Input: dimensioned drawing with shaded views. Units: mm. Origin: part minimum x, y, z. A direction names the side the tool comes from. Round coordinates to 2 decimals unless told otherwise and drop trailing zeros. Loops run counter-clockwise (first coordinate to the right, second up) from the corner with the lowest first, then second, coordinate; pieces in that order, holes last. Notation, with made-up numbers: (-13, 51) - (-1, 51) arc R22 cw to (-1, 84) - close; hole circle Ø9 at (2, 54.25). An arc over 180 degrees is marked (long way). Answer as a JSON object with one key per item and string values. Group by question number.
Item 1: Section B-B (y = 12.75). Return the cut outline in (x, z) (1 decimal), plus the area to 3 significant figures.
Item 2: Line query: line 1 (Y direction, x = 8, z = 133.5); line 2 (X direction, y = 8.5, z = 24); line 3 (Z direction, x = 15.5, y = 12.75) (1 decimal). Output: solid intervals per line, ascending.
Item 3: Reachability of the marked faces 1, 2 and 3 from +Z, -Z, +X, -X, +Y, -Y: full face, straight path, thin tool, end or side. Return the list, or none.
Item 4: Section C-C (z = 96). Return the cut outline in (x, y).
Item 5: Section D-D (y = 7). Return the cut outline in (x, z).
Item 6: First-contact query: pin 1 (1.4 mm diameter, centred on x = 6.12, z = 127.1, fed in from +Y); pin 2 (5.5 mm diameter, centred on x = 6, z = 47, fed in from +Y); pin 3 (8 mm diameter, centred on x = 8.5, y = 10, fed in from +Z); pin 4 (1.4 mm diameter, centred on x = 21.5, y = 13.5, fed in from -Z) (1 decimal). Flat tips, straight axial feed; report the tip coordinate or a pass-through.
Item 7: Section A-A (x = 39). Return the cut outline in (y, z) (1 decimal).
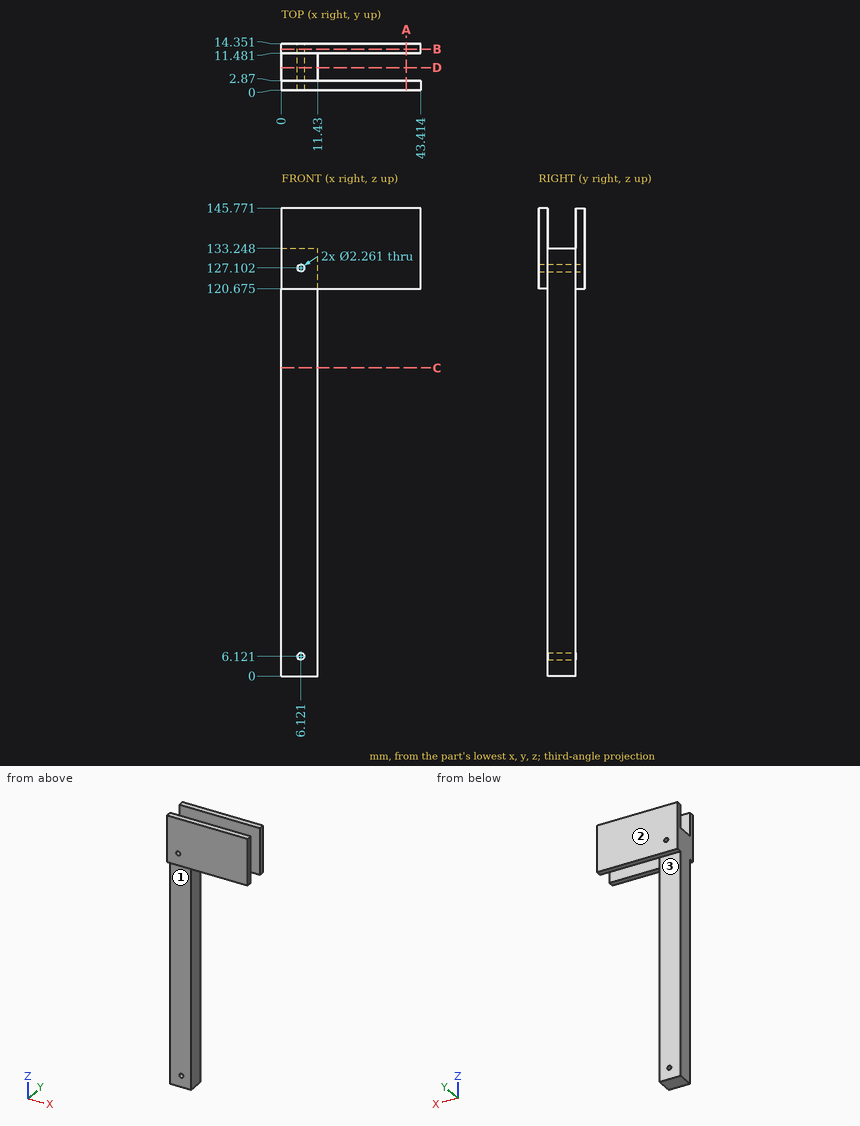
Values:
{
 "1": {"outline": "(0, 120.7) - (43.4, 120.7) - (43.4, 145.8) - (0, 145.8) - close; hole circle Ø2.3 at (6.1, 127.1)", "area": "1,090 mm^2"},
 "2": {"line 1": "y = 0 to 2.87, 11.48 to 14.35", "line 2": "x = 0 to 11.43", "line 3": "z = 120.7 to 145.8"},
 "3": {"face 1": "-Z, +X, -X, -Y", "face 2": "+Z, -Z, +X, -X, +Y", "face 3": "-Z, +X, -X, +Y"},
 "4": {"outline": "(0, 2.87) - (11.43, 2.87) - (11.43, 11.48) - (0, 11.48) - close"},
 "5": {"outline": "(0, 0) - (11.43, 0) - (11.43, 133.25) - (0, 133.25) - close; hole circle Ø2.26 at (6.12, 6.12); hole circle Ø2.26 at (6.12, 127.1)"},
 "6": {"pin 1": "passes through", "pin 2": "stops at y = 11.48", "pin 3": "stops at z = 145.77", "pin 4": "stops at z = 120.7"},
 "7": {"outline": "(0, 120.7) - (2.9, 120.7) - (2.9, 145.8) - (0, 145.8) - close; (11.5, 120.7) - (14.4, 120.7) - (14.4, 145.8) - (11.5, 145.8) - close"}
}
